The figure shows three views and two pictorial views of one solid part (mm, origin at its lowest corner). Answer the questions. Coordinates: 2 decimals unless noted, no trailing zeros. Order: outer loops, then holes, each group sorted by start corner. A loop starts at its lowest first (then second) coordinate and runs counter-clockwise, first axis right, second up. Notation, with made-up numbers: M 4.25,83.5 L 33.25,83.5 A16 ccw 33.25,105.5 Z; hole C 17,-10 d11. An arc over 180 degrees is marked long. Write item = value, one per line. Start each with the question number.
Q1. Determine the mould class of the marked faces 1 and 2 for opening direction Z: released by +Z, released by -Z, zero draft, split by the parting line, or undercut.
Q2. Find section D-D on x = 15. Give the vertices of the cut face in (y, z), and give its area (3 significant figures).
Q3. Straight lines are drawn through the part: line 1 along Z through (x, y) = (55, 15); line 2 along Y through (x, z) = (30, 2.75); line 3 along Z through (x, y) = (31.5, 56.5). For each, find the intervals that lie inside material, in ascending order.
Q4. Find section A-A on y = 30. Give the vertices of the cut face in (x, z).
Q5. Find section C-C on z = 3.75. Give the vertices of the cut face in (x, y).
Q6. Each of these flat-tipped pins is pushed along its axis until it touches: P1, Ø6, axis at x = 18.5, y = 51, coming from the +Z side; P2, Ø2.5, axis at y = 39, z = 11, coming from the +X side; P3, Ø3, axis at y = 28, z = 2.5, coming from the +X side. Where does it stop, or does it pass through?
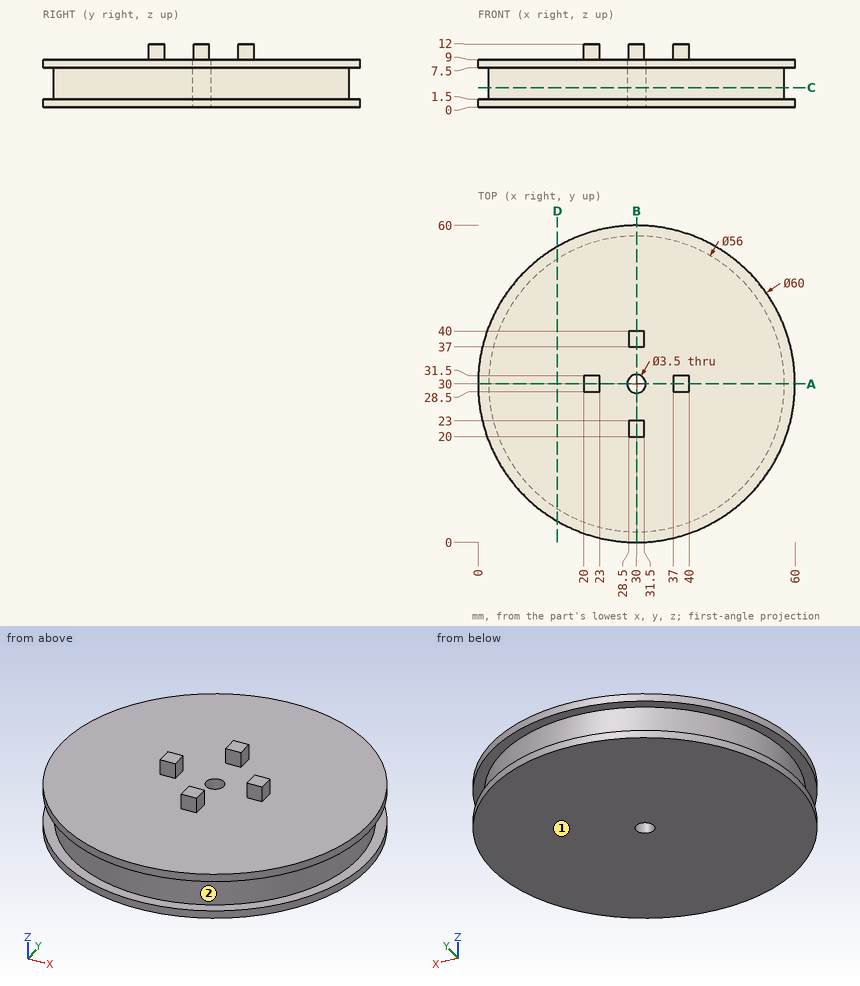
Findings below:
q1.face_1 = released by -Z
q1.face_2 = undercut
q2.outline = M 4.02,0 L 55.98,0 L 55.98,1.5 L 53.64,1.5 L 53.64,7.5 L 55.98,7.5 L 55.98,9 L 4.02,9 L 4.02,7.5 L 6.36,7.5 L 6.36,1.5 L 4.02,1.5 Z
q2.area = 440 mm^2
q3.line_1 = 0 to 1.5, 7.5 to 9
q3.line_2 = 2 to 28.25, 31.75 to 58
q3.line_3 = 0 to 9
q4.outline = M 0,0 L 28.25,0 L 28.25,9 L 23,9 L 23,12 L 20,12 L 20,9 L 0,9 L 0,7.5 L 2,7.5 L 2,1.5 L 0,1.5 Z; M 31.75,0 L 60,0 L 60,1.5 L 58,1.5 L 58,7.5 L 60,7.5 L 60,9 L 40,9 L 40,12 L 37,12 L 37,9 L 31.75,9 Z
q5.outline = C 30,30 d56; hole C 30,30 d3.5
q6.P1 = 9
q6.P2 = 31.5
q6.P3 = 59.99
